from build123d import *

# Parameters (mm, degrees)
SKETCH2_R           = 15
BOSS_EXTRUDE1_DEPTH = 10
CUT_EXTRUDE1_REACH  = 25.452
SKETCH3_R           = 5
CUT_EXTRUDE2_DEPTH  = 24.452078799


with BuildPart() as part:
    # Sketch2 → Boss-Extrude1 (new body)
    with BuildSketch(Plane.XY):
        Circle(SKETCH2_R)
    extrude(amount=BOSS_EXTRUDE1_DEPTH)

    # Sketch3 → Cut-Extrude1 (cut, up to next)
    with BuildSketch(Plane.XY.offset(10), mode=Mode.PRIVATE) as cut_extrude1_sk1:
        Circle(SKETCH3_R)
    cut_extrude1_tool1 = extrude(cut_extrude1_sk1.sketch, amount=-CUT_EXTRUDE1_REACH, mode=Mode.PRIVATE) & part.part
    add(cut_extrude1_tool1.solids().sort_by_distance((0, 0, 10))[0], mode=Mode.SUBTRACT)

    # Sketch7 → Cut-Extrude2 (cut, through all)
    with BuildSketch(Plane.XY.offset(10)):
        with BuildLine():
            ThreePointArc((3.70412729, 6.521460037), (0, 7.5), (-3.70412729, 6.521460037))
            ThreePointArc((-3.70412729, 6.521460037), (-14.165401159, 16.297297145), (0, 14.212434533))
            ThreePointArc((0, 14.212434533), (14.165401159, 16.297297145), (3.70412729, 6.521460037))
        make_face()
    extrude(amount=-CUT_EXTRUDE2_DEPTH, mode=Mode.SUBTRACT)


with BuildPart() as body_2:
    # of the pieces the cut leaves, the one that is kept (cut_extrude2_keep)
    add(part.part.solids().sort_by_distance((-12.796599287, 7.826049238, 0))[0])


solid = body_2.part
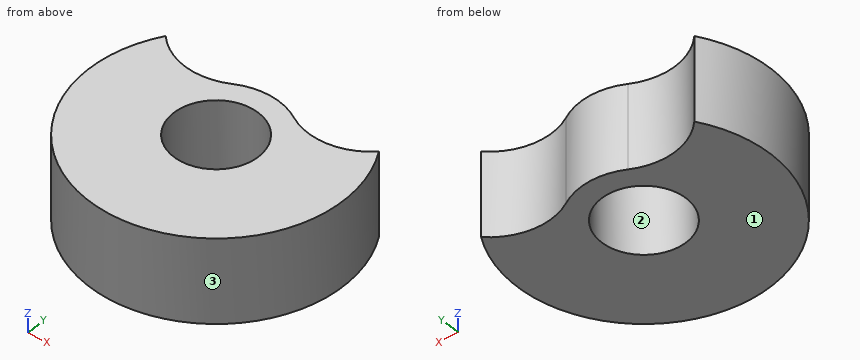
The model under review builds one solid part; all positions refer to its coordinate system, in mm. Face numbers are marked on the shaded views. Round coordinates to 2 decimals unless told otherwise and drop trailing zeros. Write each loop counter-clockwise with the first axis right and the second up, starting at its lowest first coordinate (ties: lowest second). Pieces come first, ordered by that corner, then holes. Notation, with made-up numbers: (78, -19.5) - (117, -19.5) arc R30 ccw to (117, 12.5) - close; hole circle Ø10 at (0.25, 19.5). An arc over 180 degrees is marked (long way). One line per item, written item: value. Start each with the question number.
1. Clearance check with flat-ended pins moving along their axes: P1, Ø5, axis at x = -11, z = 3, coming from the -Y side; P2, Ø8, axis at x = 0, y = 0, coming from the -Z side; P3, Ø1, axis at x = 4.5, z = 2.5, coming from the -Y side; P4, Ø5, axis at x = -5.5, z = 7.5, coming from the -Y side. State where each tip first meets the part, or that it passes through.
2. Consider section D-D on x = 7.75. Write out the cut boundary in (y, z).
3. Consider section A-A on x = 0. Write out the cut boundary in (y, z).
4. Consider section C-C on z = 4. Write out the cut boundary in (x, y), and give its area (3 significant figures).
5. To check wall thickness, follow L1, parallel to X at y = -0.25, z = 4; L2, parallel to Y at x = 3, z = 9; L3, parallel to X at y = 3.5, z = 2.25. State the ranges of each line that lie inside material, in increasing order. Write a range as from..to.
6. The part is to be moulded in two halves that separate along Y. For the marked faces 1, 2 and 3, say which applies: released by +Y, released by -Y, zero draft, split by the parting line, or undercut.
7. Consider section B-B on y = 0. Write out the cut boundary in (x, z).
Checks:
1. P1: stops at y = -12.36
1. P2: passes through
1. P3: stops at y = -14.46
1. P4: stops at y = -14.7
2. outline: (-12.84, 0) - (5.55, 0) - (5.55, 10) - (-12.84, 10) - close
3. outline: (-15, 0) - (-5, 0) - (-5, 10) - (-15, 10) - close; (5, 0) - (7.5, 0) - (7.5, 10) - (5, 10) - close
4. outline: (-12.8, 7.83) arc R15 ccw (long way) to (12.8, 7.83) arc R7.5 cw to (3.7, 6.52) arc R7.5 ccw to (-3.7, 6.52) arc R7.5 cw to start; hole circle Ø10 at (0, 0)
4. area: 462 mm^2
5. L1: x = -15..-4.99, 4.99..15
5. L2: y = -14.7..-4, 4..6.87
5. L3: x = -14.59..-3.57, 3.57..14.59
6. face 1: zero draft
6. face 2: undercut
6. face 3: split by the parting line
7. outline: (-15, 0) - (-5, 0) - (-5, 10) - (-15, 10) - close; (5, 0) - (15, 0) - (15, 10) - (5, 10) - close
